Geometry: see drawing. Coordinates: mm, zero at the bounding-box minimum. Round coordinates to 2 decimals unless told otherwise and drop trailing zeros. Loops run counter-clockwise (first coordinate to the right, second up) from the corner with the lowest first, then second, coordinate; pieces in that order, holes last. Notation, with made-up numbers: M 70,70.25 L 85,70.25 A20 ccw 85,82.25 Z; hole C -3.5,86.5 d3. An arc over 180 degrees is marked long. Answer as a JSON object with one key per item and string values.
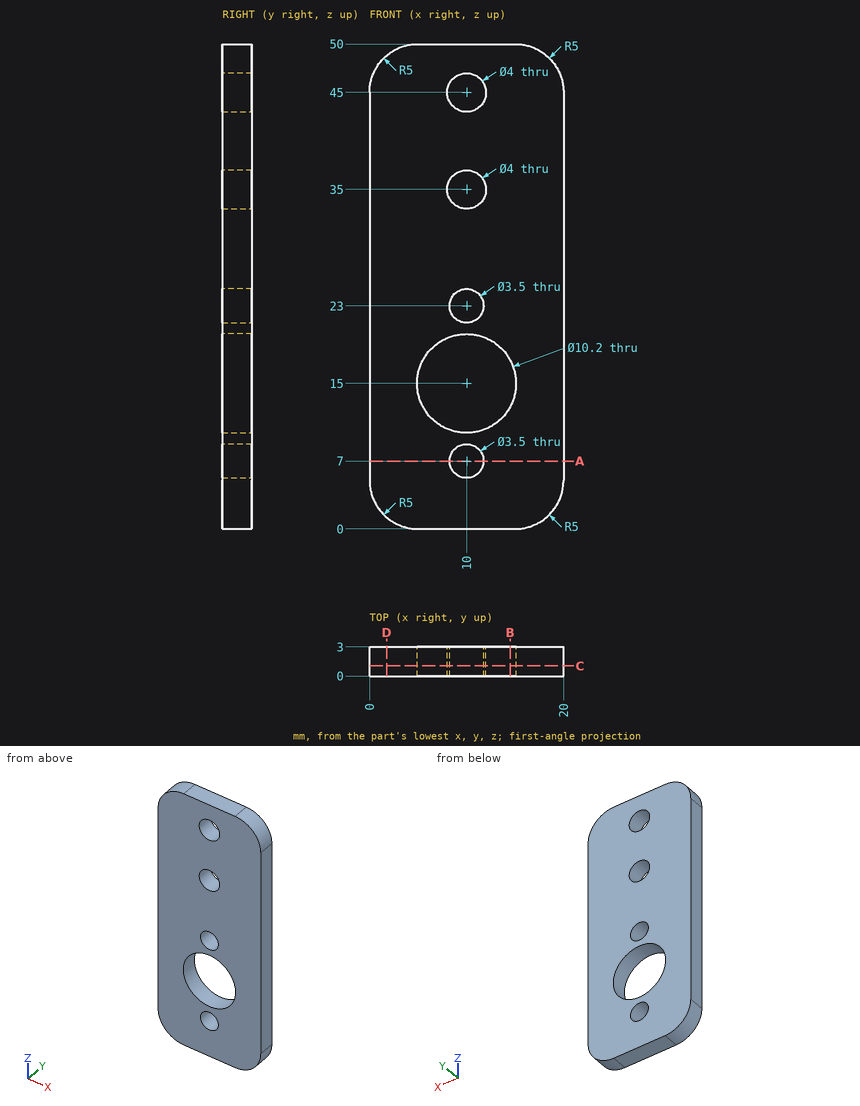
1) Section query C-C (y = 1.05). Return the cut outline in (x, z).
Results:
{"outline": "M 0,5 A5 ccw 5,0 L 15,0 A5 ccw 20,5 L 20,45 A5 ccw 15,50 L 5,50 A5 ccw 0,45 Z; hole C 10,15 d10.2; hole C 10,35 d4; hole C 10,45 d4; hole C 10,7 d3.5; hole C 10,23 d3.5"}
2) Ray query, line 1 (X direction, y = 1.15, z = 23); line 2 (X direction, y = 2.1, z = 45); line 3 (Z direction, x = 9, y = 2.35). Return the intervals inside material, ascending.
Results:
{"line 1": "0 to 8.25, 11.75 to 20", "line 2": "0 to 8, 12 to 20", "line 3": "0 to 5.56, 8.44 to 10, 20 to 21.56, 24.44 to 33.27, 36.73 to 43.27, 46.73 to 50"}
3) Section query A-A (z = 7). Return the cut outline in (x, y).
Results:
{"outline": "M 0,0 L 8.25,0 L 8.25,3 L 0,3 Z; M 11.75,0 L 20,0 L 20,3 L 11.75,3 Z"}
4) Section query B-B (x = 14.5). Return the cut outline in (y, z).
Results:
{"outline": "M 0,0 L 3,0 L 3,12.6 L 0,12.6 Z; M 0,17.4 L 3,17.4 L 3,50 L 0,50 Z"}
5) Section query D-D (x = 1.75). Return the cut outline in (y, z).
Results:
{"outline": "M 0,1.2 L 3,1.2 L 3,48.8 L 0,48.8 Z"}
